Geometry check sheet. Reference: drawing and pictorial views, mm from the part's lowest x, y, z. A direction names the side the tool comes from. Round coordinates to 2 decimals unless told otherwise and drop trailing zeros. Loops run counter-clockwise (first coordinate to the right, second up) from the corner with the lowest first, then second, coordinate; pieces in that order, holes last. Notation, with made-up numbers: (7.5, -20.75) - (39.5, -20.75) arc R16 ccw to (39.5, 7.25) - close; hole circle Ø5 at (-31.5, -21). An arc over 180 degrees is marked (long way). Answer in a Markdown table with one row per item. Add a question column.
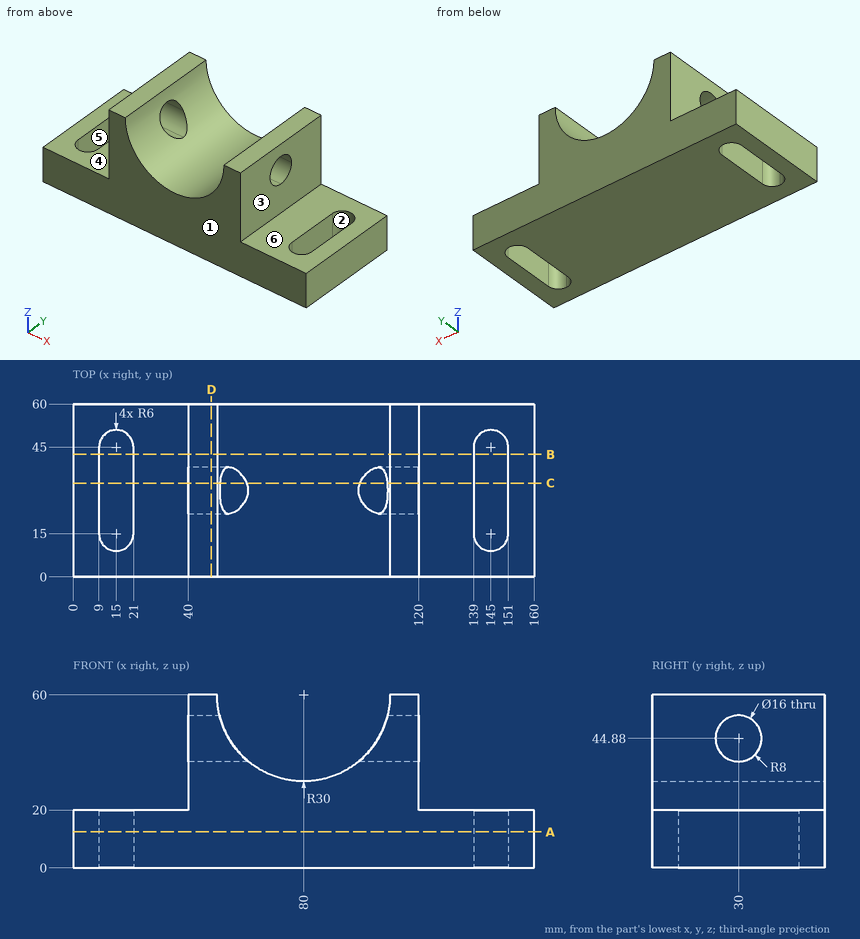
Q1. Cross-section at D-D, the plane x = 48. Enter the section's corners in (y, z), plus the area to 3 significant figures.
Q2. Cross-section at C-C, the plane y = 32.5. Enter the section's corners in (x, z), plus the area to 3 significant figures.
Q3. Cross-section at A-A, the plane z = 12.5. Enter the section's corners in (x, y).
Q4. Depth check by flat-ended pin: P1, Ø1.5, axis at x = 127, y = 50.5, coming from the +Z side; P2, Ø12, axis at y = 39.5, z = 34, coming from the +X side; P3, Ø12, axis at y = 48.5, z = 51, coming from the -X side. Enter the tip coordinate at first touch or a pass-through.
Q5. Set-up check for the marked faces 4, 5 and 6: record each of +Z, -Z, +X, -X, +Y, -Y from which the full face is reachable in a straight line by a thin tool's end or side.
Q6. Cross-section at B-B, the plane y = 42.5. Enter the section's corners in (x, z), plus the area to 3 significant figures.
Q7. Release check for a two-part mould opening along Y. For the marked faces 1, 2 and 3 record: +Y half, -Y half, draft (parallel to the pull), parting line (faces both ways), or undercut.
Q8. Scan lines: line 1 (X direction, y = 23, z = 8); line 2 (X direction, y = 11, z = 7); line 3 (Z direction, x = 79, y = 20.5). Record each from-to range of solid material in increasing order. Write a range as from..to.
Check sheet entries:
| question | item | result |
|---|---|---|
| 1 | outline | (0, 0) - (60, 0) - (60, 60) - (0, 60) - close; hole circle Ø16 at (30, 44.88) |
| 1 | area | 3,400 mm² |
| 2 | outline | (0, 0) - (9, 0) - (9, 20) - (0, 20) - close; (21, 0) - (139, 0) - (139, 20) - (120, 20) - (120, 37.28) - (99.59, 37.28) arc R30 cw to (60.41, 37.28) - (40, 37.28) - (40, 20) - (21, 20) - close; (40, 52.48) - (50.96, 52.48) arc R30 cw to (50, 60) - (40, 60) - close; (109.04, 52.48) - (120, 52.48) - (120, 60) - (110, 60) arc R30 cw to start; (151, 0) - (160, 0) - (160, 20) - (151, 20) - close |
| 2 | area | 4,060 mm² |
| 3 | outline | (0, 0) - (160, 0) - (160, 60) - (0, 60) - close; hole (9, 15) arc R6 ccw to (21, 15) - (21, 45) arc R6 ccw to (9, 45) - close; hole (139, 15) arc R6 ccw to (151, 15) - (151, 45) arc R6 ccw to (139, 45) - close |
| 4 | P1 | z = 20 |
| 4 | P2 | x = 120 |
| 4 | P3 | x = 40 |
| 5 | face 4 | +Z, -X, +Y, -Y |
| 5 | face 5 | +Z, -Z |
| 5 | face 6 | +Z, +X, +Y, -Y |
| 6 | outline | (0, 0) - (9, 0) - (9, 20) - (0, 20) - close; (21, 0) - (139, 0) - (139, 20) - (120, 20) - (120, 60) - (110, 60) arc R30 cw to (50, 60) - (40, 60) - (40, 20) - (21, 20) - close; (151, 0) - (160, 0) - (160, 20) - (151, 20) - close |
| 6 | area | 4,510 mm² |
| 7 | face 1 | -Y half |
| 7 | face 2 | undercut |
| 7 | face 3 | draft |
| 8 | line 1 | 0..9, 21..139, 151..160 |
| 8 | line 2 | 0..10.53, 19.47..140.53, 149.47..160 |
| 8 | line 3 | 0..30.02 |
